```python
from build123d import *

# Parameters (mm, degrees)
SKETCH3_W           = 60
SKETCH3_H           = 6.35
BOSS_EXTRUDE2_DEPTH = 60
SKETCH4_R           = 11.25
CUT_EXTRUDE2_DEPTH  = 7.35
SKETCH5_R           = 3.302
CUT_EXTRUDE3_DEPTH  = 7.35
CUT_EXTRUDE4_DEPTH  = 7.35


with BuildPart() as part:
    # Sketch3 → Boss-Extrude2 (new body)
    with BuildSketch(Plane.XY):
        with Locations((30, 3.175)):
            Rectangle(SKETCH3_W, SKETCH3_H)
    extrude(amount=BOSS_EXTRUDE2_DEPTH)

    # Sketch4 → Cut-Extrude2 (cut, through all)
    with BuildSketch(Plane(origin=(0, 6.35, 0), x_dir=(1, 0, 0), z_dir=(0, 1, 0))):
        with Locations((30, -30)):
            Circle(SKETCH4_R)
    extrude(amount=-CUT_EXTRUDE2_DEPTH, mode=Mode.SUBTRACT)

    # Sketch5 → Cut-Extrude3 (cut, through all)
    with BuildSketch(Plane(origin=(0, 6.35, 0), x_dir=(1, 0, 0), z_dir=(0, 1, 0))):
        with Locations((20.658415592, -6.810890471)):
            Circle(SKETCH5_R)
        with Locations((49.167445389, -13.949796348)):
            Circle(SKETCH5_R)
        with Locations((51.187717135, -43.269538146)):
            Circle(SKETCH5_R)
        with Locations((23.927283945, -54.251229241)):
            Circle(SKETCH5_R)
        with Locations((5.059137939, -31.718545794)):
            Circle(SKETCH5_R)
    extrude(amount=-CUT_EXTRUDE3_DEPTH, mode=Mode.SUBTRACT)

    # Sketch6 → Cut-Extrude4 (cut, through all)
    with BuildSketch(Plane(origin=(0, 6.35, 0), x_dir=(1, 0, 0), z_dir=(0, 1, 0))):
        with BuildLine():
            ThreePointArc((0, -30), (8.786796564, -8.786796564), (30, 0))
            Line((30, 0), (0, 0))
            Line((0, 0), (0, -30))
        make_face()
        with BuildLine():
            Line((60, -30), (60, 0))
            Line((60, 0), (30, 0))
            ThreePointArc((30, 0), (51.213203436, -8.786796564), (60, -30))
        make_face()
        with BuildLine():
            Line((60, -60), (60, -30))
            ThreePointArc((60, -30), (51.213203436, -51.213203436), (30, -60))
            Line((30, -60), (60, -60))
        make_face()
        with BuildLine():
            ThreePointArc((30, -60), (8.786796564, -51.213203436), (0, -30))
            Line((0, -30), (0, -60))
            Line((0, -60), (30, -60))
        make_face()
    extrude(amount=-CUT_EXTRUDE4_DEPTH, mode=Mode.SUBTRACT)


solid = part.part
```
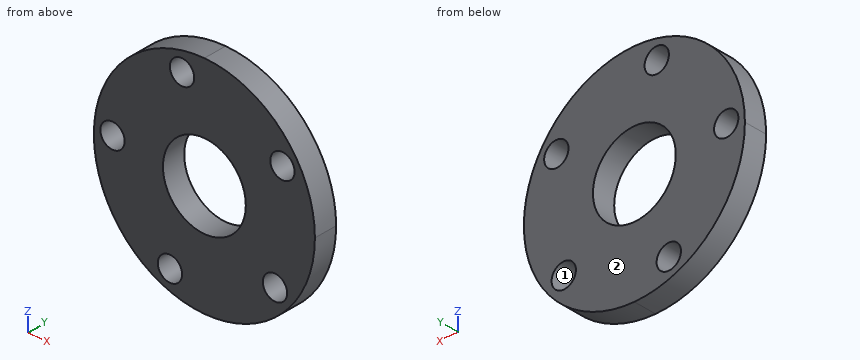
Geometry: final body of the model. Coordinates: model frame, mm. Face numbers are marked on the shaded views. Give positions to 0.01 mm unless a question says otherwise; leave off trailing zeros. Loops run counter-clockwise (first coordinate to the right, second up) from the corner with the lowest first, then second, coordinate; pieces in that order, holes last. Notation, with made-up numbers: (-28.75, 12) -> (15.25, 12) arc R24 cw to (15.25, 48) -> close; hole circle Ø11 at (50.25, -12). An arc over 180 degrees is marked (long way). Use one line per item in the form item = value.
Item 1: Pin query (flat end, axial travel): P1, Ø10, axis at x = 36.5, z = 15, coming from the -Y side; P2, Ø5.5, axis at x = 23.93, z = 54.25, coming from the +Y side; P3, Ø1, axis at y = 5.5, z = 21, coming from the +X side; P4, Ø2, axis at y = 2.5, z = 27.5, coming from the -X side. Return the tip coordinate at first contact, or that it passes through.
A:
P1 = 0
P2 = through
P3 = 58.77
P4 = 0.04
Item 2: Line query: probe 1 along Z at (x, y) = (30, 3); probe 2 along Z at (x, y) = (24, 0.5); probe 3 along Z at (x, y) = (23, 1.5). Output: solid intervals per line, ascending.
A:
probe_1 = 0 to 18.75, 41.25 to 60
probe_2 = 0.61 to 20.48, 39.52 to 50.95, 57.55 to 59.39
probe_3 = 0.83 to 4.48, 9.14 to 21.19, 38.81 to 51.08, 57.42 to 59.17
Item 3: Section query B-B on x = 31. Output: boundary loops of the cut face in (y, z).
A:
outline = (0, 0.02) -> (6.35, 0.02) -> (6.35, 18.79) -> (0, 18.79) -> close; (0, 41.21) -> (6.35, 41.21) -> (6.35, 59.98) -> (0, 59.98) -> close
Item 4: Section query A-A on z = 27. Output: boundary loops of the cut face in (x, y), and give its area (3 significant figures).
A:
outline = (0.15, 0) -> (19.16, 0) -> (19.16, 6.35) -> (0.15, 6.35) -> close; (40.84, 0) -> (59.85, 0) -> (59.85, 6.35) -> (40.84, 6.35) -> close
area = 241 mm^2
Item 5: Section query C-C on y = 2. Output: boundary loops of the cut face in (x, z), and give its area (3 significant figures).
A:
outline = circle Ø60 at (30, 30); hole circle Ø6.6 at (5.06, 31.72); hole circle Ø6.6 at (20.66, 6.81); hole circle Ø22.5 at (30, 30); hole circle Ø6.6 at (23.93, 54.25); hole circle Ø6.6 at (49.17, 13.95); hole circle Ø6.6 at (51.19, 43.27)
area = 2,260 mm^2
Item 6: Section query D-D on z = 33. Output: boundary loops of the cut face in (x, y), and give its area (3 significant figures).
A:
outline = (0.15, 0) -> (2.02, 0) -> (2.02, 6.35) -> (0.15, 6.35) -> close; (8.1, 0) -> (19.16, 0) -> (19.16, 6.35) -> (8.1, 6.35) -> close; (40.84, 0) -> (59.85, 0) -> (59.85, 6.35) -> (40.84, 6.35) -> close
area = 203 mm^2
Item 7: Draft query along X for the marked faces 1 and 2. Return one class per face: pulls with the +X half, pulls with the -X half, needs draft (parallel to the pull), parting line crosses it, or undercut.
A:
face_1 = undercut
face_2 = needs draft
